```python
from build123d import *

# Parameters (mm, degrees)
SKETCH1_W           = 55
SKETCH1_H           = 45
BOSS_EXTRUDE1_DEPTH = 3
SKETCH2_W           = 10
SKETCH2_H           = 13
BOSS_EXTRUDE2_DEPTH = 12.5
SKETCH3_R           = 1.75
CUT_EXTRUDE1_DEPTH  = 13.5
FILLET1_R           = 6
CHAMFER1_SIZE       = 12
FILLET3_R           = 1
SKETCH4_W           = 20
SKETCH4_H           = 10
CUT_EXTRUDE3_DEPTH  = 5
SKETCH7_R           = 1.75
CUT_EXTRUDE4_DEPTH  = 5
BOSS_EXTRUDE4_DEPTH = 3


with BuildPart() as part:
    # Sketch1 → Boss-Extrude1 (new body)
    with BuildSketch(Plane.XY):
        with Locations((-16.936997319, -3.156836461)):
            Rectangle(SKETCH1_W, SKETCH1_H)
    extrude(amount=BOSS_EXTRUDE1_DEPTH)

    # Sketch2 → Boss-Extrude2 (add)
    with BuildSketch(Plane(origin=(0, 0, 0), x_dir=(-1, 0, 0), z_dir=(0, 0, -1))):
        with Locations((-5.563002681, -3.156836461)):
            Rectangle(SKETCH2_W, SKETCH2_H)
    extrude(amount=BOSS_EXTRUDE2_DEPTH)

    # Sketch3 → Cut-Extrude1 (cut)
    with BuildSketch(Plane(origin=(0, 3.343163539, 0), x_dir=(1, 0, 0), z_dir=(0, 1, 0))):
        with Locations(Location((5.563002681, 7.5, 0), (0, 0, 180))):
            Circle(SKETCH3_R)
    extrude(amount=-CUT_EXTRUDE1_DEPTH, mode=Mode.SUBTRACT)

    # Fillet1
    fillet1_edges = [part.edges().sort_by_distance(p)[0] for p in [
        (10.563002681, -3.156836461, -12.5),
    ]]
    fillet(fillet1_edges, radius=FILLET1_R)

    # Chamfer1
    chamfer1_edges = [part.edges().sort_by_distance(p)[0] for p in [
        (0.563002681, -3.156836461, 0),
    ]]
    chamfer(chamfer1_edges, length=CHAMFER1_SIZE)

    # Fillet3
    # the kernel refuses this fillet: 1 mm, written as the material it takes off along each edge
    with BuildSketch(Plane(origin=(0.563002681, 5.508227048, -12.5), x_dir=(1, 0, 0), z_dir=(0, -1, 0))) as fillet3_piece_1:
        with BuildLine():
            CenterArc((0.866025404, 1), FILLET3_R, 210, 60)
            Line((0, 0.5), (-0.017320508, 0.49))
            ThreePointArc((-0.017320508, 0.49), (-0.02, 0.25), (-0.02, 0))
            Line((-0.02, 0), (0, -0.02))
            Line((0, -0.02), (0.866025404, -0.02))
            Line((0.866025404, -0.02), (0.866025404, 0))
        make_face()
    extrude(amount=17.330127019, mode=Mode.SUBTRACT)

    # Sketch4 → Cut-Extrude3 (cut)
    with BuildSketch(Plane(origin=(0, 0, 0), x_dir=(-1, 0, 0), z_dir=(0, 0, -1))):
        with Locations((-5.563002681, 8.343163539)):
            Rectangle(SKETCH4_W, SKETCH4_H)
    cut_extrude3 = extrude(amount=-CUT_EXTRUDE3_DEPTH, mode=Mode.SUBTRACT)

    # Mirror2: Cut-Extrude3 across plane
    add(cut_extrude3.mirror(Plane.ZX.offset(-3.156836461)), mode=Mode.SUBTRACT)

    # Sketch7 → Cut-Extrude4 (cut)
    with BuildSketch(Plane(origin=(0, 0, 0), x_dir=(-1, 0, 0), z_dir=(0, 0, -1))):
        with Locations((-1.563002681, 16.343163539)):
            Circle(SKETCH7_R)
        with Locations((39.436997319, 16.343163539)):
            Circle(SKETCH7_R)
        with Locations(Location((39.436997319, -22.656836461, 0), (0, 0, 180))):
            Circle(SKETCH7_R)
        with Locations(Location((-1.563002681, -22.656836461, 0), (0, 0, 180))):
            Circle(SKETCH7_R)
    extrude(amount=-CUT_EXTRUDE4_DEPTH, mode=Mode.SUBTRACT)

    # Sketch8 → Boss-Extrude4 (add)
    with BuildSketch(Plane(origin=(0, 0, 0), x_dir=(-1, 0, 0), z_dir=(0, 0, -1))):
        Polygon((44.436997319, 6.843163539), (51.936997319, 6.843163539), (51.936997319, 9.343163539), (59.436997319, 4.091607002), (59.436997319, -10.405279925), (51.936997319, -15.656836461), (51.936997319, -13.156836461), (44.436997319, -13.156836461), align=None)
    extrude(amount=-BOSS_EXTRUDE4_DEPTH)


solid = part.part
```
Geometry: final body of the model. Coordinates: model frame, mm. A direction names the side the tool comes from. Give positions to 0.01 mm unless a question says otherwise; leave off trailing zeros. Write each loop counter-clockwise with the first axis right and the second up, starting at its lowest first coordinate (ties: lowest second). Pieces come first, ordered by that corner, then holes.
1. Line query: probe 1 along Y at (x, z) = (-3, -5.5); probe 2 along Z at (x, y) = (-49.5, -6); probe 3 along Z at (x, y) = (5, -5). Output: solid intervals per line, ascending.
2. Section query D-D, the plane x = -17. Return loops of the section in (y, z), then the cut area to 3 significant figures.
3. Section query A-A, the plane y = -3. Return loops of the section in (x, z), then the cut area to 3 significant figures.
4. Section query C-C, the plane x = -40. Return loops of the section in (y, z), then the cut area to 3 significant figures.
5. Draft query along X for faces 1 (the cylindrical face through (8.85, -3.07, -10.7)), 2 (the flat face through (-17, -25.657, 1)), 3 (the flat face through (-51.937, 8, 1)), 4 (the cylindrical face through (1.335, -24.392, 1.479)). Return one class per face: released by +X, released by -X, zero draft, split by the parting line, or undercut.
6. Section query B-B, the plane z = -7.5. Return loops of the section in (x, y).
7. Reachability of faces 5 (the flat face through (-44.437, 13, 1)), 6 (the flat face through (3, 13.343, 1)), 7 (the flat face through (-51.937, -14, 1)) from +Z, -Z, +X, -X, +Y, -Y: full face, straight path, thin tool, end or side. Return the list, or none.
8. Pin query (flat end, axial travel): P1, Ø3.5, axis at x = -48, z = 2, coming from the +Y side; P2, Ø4, axis at x = -39.44, y = 16.34, coming from the -Z side; P3, Ø2, axis at y = -15, z = 2, coming from the +X side. Return the tip coordinate at first contact, or that it passes through.
Computed:
1. probe 1: y = -9.66 to 3.34
1. probe 2: z = 0 to 3
1. probe 3: z = -12.48 to -9.16, -5.84 to 3
2. outline: (-25.66, 0) - (19.34, 0) - (19.34, 3) - (-25.66, 3) - close
2. area: 135 mm2
3. outline: (-59.44, 0) - (-11.44, 0) - (0.56, -12) arc R1 ccw to (1.43, -12.5) - (4.56, -12.5) arc R6 ccw to (10.56, -6.5) - (10.56, 3) - (-59.44, 3) - close; hole circle Ø3.5 at (5.56, -7.5)
3. area: 390 mm2
4. outline: (-25.66, 0) - (-24.31, 0) - (-24.31, 3) - (-25.66, 3) - close; (-21, 0) - (14.69, 0) - (14.69, 3) - (-21, 3) - close; (18, 0) - (19.34, 0) - (19.34, 3) - (18, 3) - close
4. area: 115 mm2
5. face 1: released by +X
5. face 2: zero draft
5. face 3: undercut
5. face 4: undercut
6. outline: (-3.94, -9.66) - (3.81, -9.66) - (3.81, 3.34) - (-3.94, 3.34) - close; (7.31, -9.66) - (10.48, -9.66) - (10.48, 3.34) - (7.31, 3.34) - close
7. face 5: +Z, -Z, +Y
7. face 6: +Z, -Z, +X
7. face 7: +Z, -Z, -Y
8. P1: stops at y = 6.84
8. P2: stops at z = 0
8. P3: stops at x = -4.44
